For this review, use the dimensioned drawing (mm, ordinates from the lowest corner) and the shaded views. Coordinates: 2 decimals unless noted, no trailing zeros. Order: outer loops, then holes, each group sorted by start corner. A loop starts at its lowest first (then second) coordinate and runs counter-clockwise, first axis right, second up. Notation, with made-up numbers: M 70,15.25 L 75,15.25 A33 cw 75,46.25 Z; hole C -16.75,17 d7. An arc over 180 degrees is marked long. One line per item, written item: value.
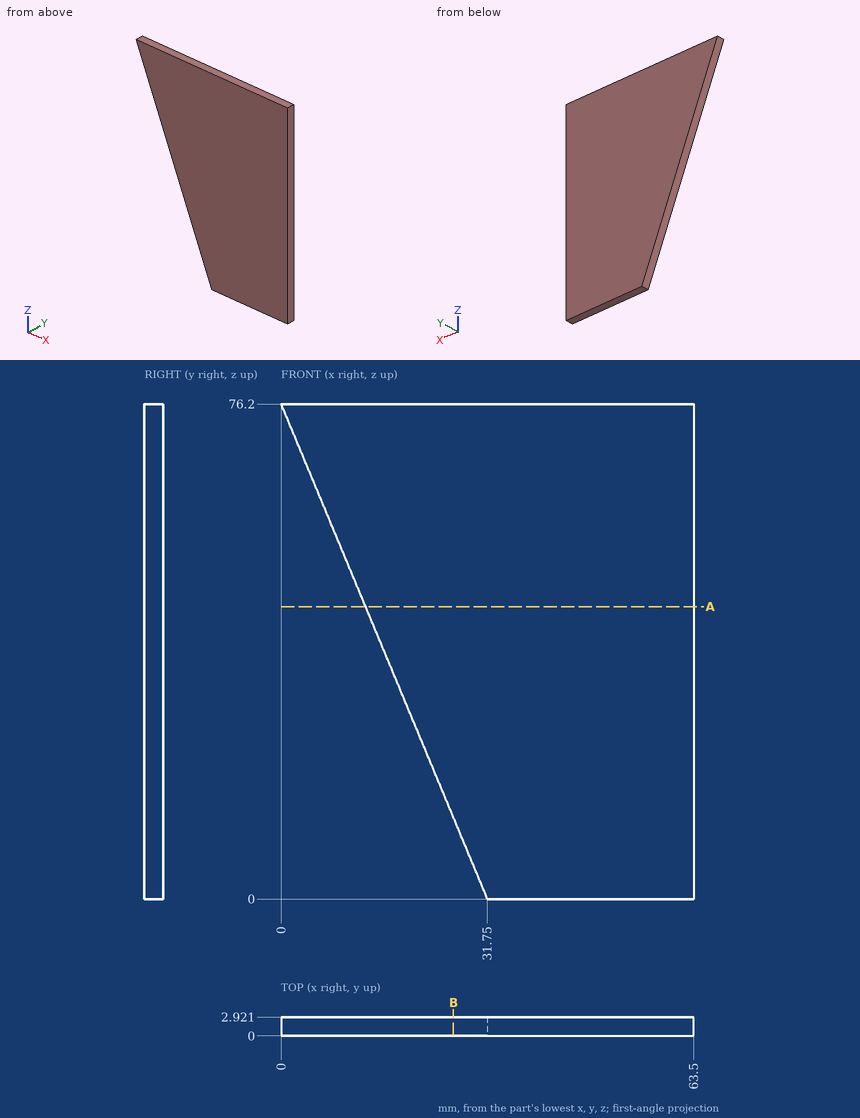
(1) We need section A-A, the plane z = 45. State the section outline as (x, y) points, plus the area to 3 significant figures.
Geometry results:
outline: M 13,0 L 63.5,0 L 63.5,2.92 L 13,2.92 Z
area: 148 mm2
(2) For L1, parallel to X at y = 1.15, z = 54; L2, parallel to X at y = 2.55, z = 67; L3, parallel to Z at x = 13, y = 2.2, list the stretches that pass through material, from the lowest coordinate up.
Geometry results:
L1: x = 9.25 to 63.5
L2: x = 3.83 to 63.5
L3: z = 45 to 76.2
(3) Insertion check: pin 1 Ø1 at (x, y) = (19.5, 2) entering from -Z. The pin has a flat end and moves straight along its axis. Give the tip position at first contact, or say it passes through.
Geometry results:
pin 1: stops at z = 28.2
(4) We need section B-B, the plane x = 26.5. State the section outline as (y, z) points.
Geometry results:
outline: M 0,12.6 L 2.92,12.6 L 2.92,76.2 L 0,76.2 Z
